from build123d import *

# Parameters (mm, degrees)
F0_W     = 62.345456332
F0_H     = 34.5733892173
F1_DEPTH = 25
F2_W     = 40.1466805488
F2_H     = 17.7154000849
F3_DEPTH = 15
F3_TAPER = 3
F4_R     = 3


with BuildPart() as f1:
    # F0 (on Top) → F1 (new body)
    with BuildSketch(Plane.XY):
        with Locations((0, -0.1889253035)):
            Rectangle(F0_W, F0_H)
    extrude(amount=-F1_DEPTH)

    # F2 (on face) → F3 (cut)
    with BuildSketch(Plane.XY):
        with Locations((0.5009016022, 0.604307279)):
            Rectangle(F2_W, F2_H)
    extrude(amount=-F3_DEPTH, taper=F3_TAPER, mode=Mode.SUBTRACT)

    # F4
    f4_edges = [f1.edges().sort_by_distance(p)[0] for p in [
        (-19.17938, 9.068949, -7.5),
        (-19.17938, -7.860334, -7.5),
        (20.181184, 9.068949, -7.5),
        (20.181184, -7.860334, -7.5),
    ]]
    fillet(f4_edges, radius=F4_R)


solid = f1.part
Could you check a few things on this model? Use its own coordinates, in mm. Give positions to 0.01 mm unless a question says otherwise; leave off trailing zeros. Return JSON: item names as keys, results as strings.
1. For pin 1 Ø8 at (x, y) = (10, -0.5) entering from +Z, with a flat end and sliding along its axis, tell me the tip position at first contact or that it passes through.
Answer list:
{"pin 1": "stops at z = -15"}
2. Thinking about a two-plate mould opening in Y: for faces 1 (the flat face through (0, 17.098, -12)), 2 (the flat face through (0, 12, 0)), 3 (the flat face through (0, 1, -15)), which applies, pulls with the +Y half, pulls with the -Y half, needs draft (parallel to the pull), parting line crosses it, or undercut?
Answer list:
{"face 1": "pulls with the +Y half", "face 2": "needs draft", "face 3": "undercut"}
3. I need wall thicknesses on line 1 (Y direction, x = 17.5, z = -6); line 2 (X direction, y = 7.5, z = -3.25); line 3 (Y direction, x = -8.5, z = -3.5). Which ranges of each line are inside material? Lowest first, please. Write a range as from..to.
Answer list:
{"line 1": "y = -17.48..-7.93, 9.14..17.1", "line 2": "x = -31.17..-19.15, 20.15..31.17", "line 3": "y = -17.48..-8.07, 9.28..17.1"}
